Read the model definition and answer for the solid it produces. Units are mm, in the model's axes. Face numbers are marked on the shaded views. Give positions to 0.01 mm unless a question says otherwise; leave off trailing zeros. Write each loop counter-clockwise with the first axis right and the second up, starting at its lowest first coordinate (ties: lowest second). Pieces come first, ordered by that corner, then holes. Notation, with made-up numbers: M 80,30 L 133,30 A14 ccw 133,52 Z; hole C 41,54 d7. An arc over 180 degrees is marked long. Use a Markdown table: item, result. Add a question column.
Item 1: A cutting plane is placed at A-A on z = 3. Determine the outline of the cut face in (x, y), then the cut area to 3 significant figures.
Item 2: The mould has two halves that part along Y. Classify the marked faces 1, 2 and 3: pulls with the +Y half, pulls with the -Y half, needs draft (parallel to the pull), parting line crosses it, or undercut.
Item 3: Given P1, Ø1, axis at y = -0.5, z = 7.5, coming from the +X side; P2, Ø1.5, axis at y = -0.5, z = 7.5, coming from the +X side, each flat-ended and moving along its own axis, determine where each tip first touches the part or whether it passes through.
Item 4: A cutting plane is placed at B-B on x = -0.3. Determine the outline of the cut face in (y, z).
Item 5: A cutting plane is placed at C-C on y = 0. Determine the outline of the cut face in (x, z), then the cut area to 3 significant figures.
Item 6: Consider probe 1 along X at (y, z) = (0.3, 2.5); probe 2 along X at (y, z) = (-0.95, 3.5); probe 3 along Y at (x, z) = (0, 5.75). Determine where each line is inside the solid, lowest interval first. Write a range as [from, to].
from build123d import *

# Parameters (mm, degrees)
SKETCH1_R           = 1.75
SKETCH1_R_2         = 1.25
BOSS_EXTRUDE1_DEPTH = 12
CUT_EXTRUDE2_START  = -12
CUT_EXTRUDE2_DEPTH  = 12


with BuildPart() as part:
    # Sketch1 → Boss-Extrude1 (new body)
    with BuildSketch(Plane.XY):
        Circle(SKETCH1_R)
        Circle(SKETCH1_R_2, mode=Mode.SUBTRACT)
    extrude(amount=BOSS_EXTRUDE1_DEPTH)

    # Sketch2 → Cut-Extrude2 (cut)
    with BuildSketch(Plane.XY.offset(12).offset(CUT_EXTRUDE2_START)):
        with BuildLine():
            ThreePointArc((-1.09434695, 1.365615156), (-1.630539837, 0.635483942), (-1.729830892, -0.264924681))
            Line((-1.729830892, -0.264924681), (-1.09434695, 1.365615156))
        make_face()
        with BuildLine():
            Line((-1.09434695, 1.365615156), (0.635483942, 1.630539837))
            ThreePointArc((0.635483942, 1.630539837), (-0.264924681, 1.729830892), (-1.09434695, 1.365615156))
        make_face()
        with BuildLine():
            Line((0.635483942, 1.630539837), (1.729830892, 0.264924681))
            ThreePointArc((1.729830892, 0.264924681), (1.365615156, 1.09434695), (0.635483942, 1.630539837))
        make_face()
        with BuildLine():
            Line((1.729830892, 0.264924681), (1.09434695, -1.365615156))
            ThreePointArc((1.09434695, -1.365615156), (1.577594238, -0.757427501), (1.75, 0))
            ThreePointArc((1.75, 0), (1.744950438, 0.132845662), (1.729830892, 0.264924681))
        make_face()
        with BuildLine():
            ThreePointArc((-0.635483942, -1.630539837), (0.264924681, -1.729830892), (1.09434695, -1.365615156))
            Line((1.09434695, -1.365615156), (-0.635483942, -1.630539837))
        make_face()
        with BuildLine():
            ThreePointArc((-1.729830892, -0.264924681), (-1.365615156, -1.09434695), (-0.635483942, -1.630539837))
            Line((-0.635483942, -1.630539837), (-1.729830892, -0.264924681))
        make_face()
    extrude(amount=CUT_EXTRUDE2_DEPTH, mode=Mode.SUBTRACT)


solid = part.part
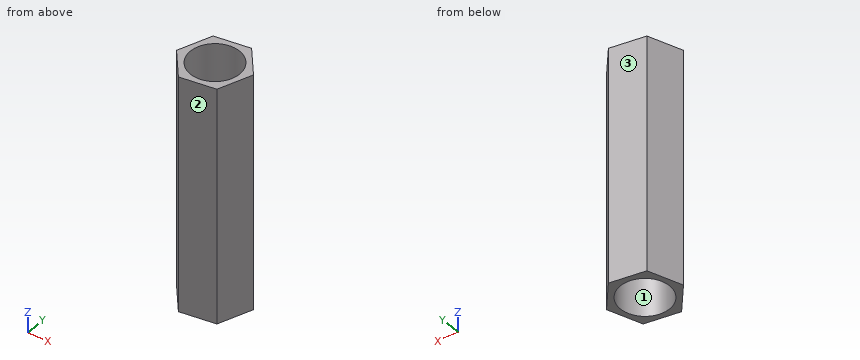
Filled in:
| question | item | result |
|---|---|---|
| 1 | outline | M -1.73,-0.26 L -0.64,-1.63 L 1.09,-1.37 L 1.73,0.26 L 0.64,1.63 L -1.09,1.37 Z; hole C 0,0 d2.5 |
| 1 | area | 3.05 mm² |
| 2 | face 1 | undercut |
| 2 | face 2 | pulls with the -Y half |
| 2 | face 3 | pulls with the +Y half |
| 3 | P1 | x = 1.63 |
| 3 | P2 | x = 1.72 |
| 4 | outline | M -1.58,0 L -1.21,0 L -1.21,12 L -1.58,12 Z; M 1.21,0 L 1.49,0 L 1.49,12 L 1.21,12 Z |
| 5 | outline | M -1.63,0 L -1.25,0 L -1.25,12 L -1.63,12 Z; M 1.25,0 L 1.63,0 L 1.63,12 L 1.25,12 Z |
| 5 | area | 9.04 mm² |
| 6 | probe 1 | [-1.51, -1.21], [1.21, 1.7] |
| 6 | probe 2 | [-1.18, -0.81], [0.81, 1.26] |
| 6 | probe 3 | [-1.53, -1.25], [1.25, 1.53] |
